Autodesk Inventor part; units mm, degrees
ref_plane "Work Plane1" through (0, 130, 0) normal (0, 1, 0) x (-1, 0, 0)
ref_plane "Work Plane2" through (0, 0, 24.9) normal (0, 0, -1) x (-1, 0, 0)
ref_plane "YZ Plane" through (0, 0, 0) normal (1, 0, 0) x (0, 1, 0)
sketch "Sketch1" plane through (0, 0, 0) normal (0, 0, 1) x (1, 0, 0)
  line L0 (-24.9, 127.5931) -> (-24.9, 125)
  line L1 (-24.9, 125) -> (24.9, 125)
  line L2 (24.9, 125) -> (24.9, 127.5931)
  arc A0 (24.9, 127.5931) -> (-24.9, 127.5931) centre (0, 0) ccw
  point P0 (0, 130)
  dimension "d0" = 130
  dimension "d1" = 5
  dimension "d2" = 49.8
extrude "Extrusion1" add sketch "Sketch1" along normal blind 49.8
chamfer "Chamfer1" distance 5 angle 45 1 edges at (-24.9, 126.2965, 49.8)
ref_plane "Work Plane1" through (0, 130, 0) normal (0, 1, 0) x (-1, 0, 0)
sketch "Sketch2" plane through (0, 130, 0) normal (0, 1, 0) x (-1, 0, 0)
  line L0 (19.9, 49.8) -> (-24.9, 49.8) construction
  line L1 (-24.9, 0) -> (-24.9, 49.8) construction
  line L2 (-24.9, 24.9) -> (31.0612, 24.9) construction
  line L3 (21.9246, 24.9) -> (17.7633, 29.1517)
  line L4 (17.7633, 29.1517) -> (17.7633, 26.5283)
  line L5 (17.7633, 26.5283) -> (13.964, 26.5283)
  line L6 (13.964, 26.5283) -> (13.964, 24.9)
  line L7 (21.9246, 24.9) -> (17.7633, 20.6483)
  line L8 (17.7633, 20.6483) -> (17.7633, 23.2717)
  line L9 (17.7633, 23.2717) -> (13.964, 23.2717)
  line L10 (13.964, 23.2717) -> (13.964, 24.9)
  point P0 (0, 0)
emboss "Emboss1" sketch "Sketch2" operation cut depth 0.8 direction (0, -1, 0)
sketch "Sketch3" plane through (-24.9, 125, 0) normal (0, -1, 0) x (1, 0, 0)
  line L0 (0, 0) -> (49.8, 0)
  line L1 (49.8, 0) -> (49.8, 49.8) construction
  line L2 (49.8, 24.9) -> (6.096, 24.9) construction
  circle A0 centre (18.3, 4.9) radius 3.5
  circle A1 centre (37.55, 4.9) radius 3.5
  circle A2 centre (18.3, 12.4) radius 2.75
  point P0 (24.9, 0)
  dimension "d20" = 7
  dimension "d21" = 7
  dimension "d22" = 20
  dimension "d23" = 20
  dimension "d24" = 12.25
  dimension "d25" = 19.25
  dimension "d26" = 5.5
  dimension "d27" = 12.5
extrude "Extrusion2" cut sketch "Sketch3" against normal blind 2.5
ref_plane "Work Plane2" through (0, 0, 24.9) normal (0, 0, -1) x (-1, 0, 0)
mirror "Mirror1" about plane through (0, 0, 24.9) normal (0, 0, -1) of "Extrusion2"
properties part number "power_signal_socket_cap"
Check sheet for the modelled part. Datum: model origin and axes. Units: mm. A direction names the side the tool comes from. Give positions to 0.01 mm unless a question says otherwise; leave off trailing zeros. Loops run counter-clockwise (first coordinate to the right, second up) from the corner with the lowest first, then second, coordinate; pieces in that order, holes last. Notation, with made-up numbers: M 71,-26 L 104,-26 A17 cw 104,-21 Z; hole C 11.5,61.5 d11. An arc over 180 degrees is marked long. Return JSON: item names as keys, results as strings. Group by question number.
1. Cross-section at A-A on y = 126.25. Record the boundary of the cut face in (x, z), plus the area to 3 significant figures.
2. Thickness scan on L1, parallel to Z at x = -6.6, y = 126.75; L2, parallel to X at y = 126.2, z = 44.5; L3, parallel to X at y = 125.85, z = 44.9. Record the ranges inside material, lowest first.
3. Cross-section at D-D on x = 12.65. Record the boundary of the cut face in (y, z), plus the area to 3 significant figures.
4. Cross-section at C-C on z = 12.4. Record the boundary of the cut face in (x, y).
5. Mould release check, pull along Z, two halves, no side actions. Record for faces 1 (the flat face through (2, 128, 49.8)), 2 (the flat face through (-7, 127.5, 5)), 3 (the flat face through (-24.9, 126, 22)): released by +Z, released by -Z, zero draft, split by the parting line, or undercut.
6. Tool access check on faces 4 (the cylindrical face through (0, 130, 25)), 5 (the flat face through (-15.9, 128.6, 26.528)), 6 (the flat face through (-7, 127.5, 37)). Record the directions out of +Z, -Z, +X, -X, +Y, -Y that give a thin tool (end or side, any length) a straight path to the whole face; none if there is none.
7. Go/stop test with flat-tipped pins: pin 1 (5 mm diameter, centred on x = -6.6, z = 12.4, fed in from -Y); pin 2 (5.5 mm diameter, centred on x = -7.5, z = 43.5, fed in from -Y); pin 3 (8 mm diameter, centred on x = 12.65, z = 4.9, fed in from +Y). Record where each tip stops, or that it passes through.
8. Cross-section at B-B on x = -7.5. Record the boundary of the cut face in (y, z).
Return value:
{
 "1": {"outline": "M -24.9,0 L 24.9,0 L 24.9,49.8 L -19.9,49.8 L -24.9,44.8 Z; hole C -6.6,4.9 d7; hole C -6.6,44.9 d7; hole C -6.6,12.4 d5.5; hole C -6.6,37.4 d5.5; hole C 12.65,4.9 d7; hole C 12.65,44.9 d7", "area": "2,270 mm^2"},
 "2": {"L1": "0 to 1.4, 8.4 to 9.65, 15.15 to 34.65, 40.15 to 41.4, 48.4 to 49.8", "L2": "-24.9 to -10.08, -3.12 to 9.17, 16.13 to 24.9", "L3": "-24.8 to -10.1, -3.1 to 9.15, 16.15 to 24.9"},
 "3": {"outline": "M 125,0 L 129.38,0 L 129.38,49.8 L 125,49.8 L 125,48.4 L 127.5,48.4 L 127.5,41.4 L 125,41.4 L 125,8.4 L 127.5,8.4 L 127.5,1.4 L 125,1.4 Z", "area": "183 mm^2"},
 "4": {"outline": "M -24.9,125 L -9.35,125 L -9.35,127.5 L -3.85,127.5 L -3.85,125 L 24.9,125 L 24.9,127.59 A130 ccw -24.9,127.59 Z"},
 "5": {"face 1": "released by +Z", "face 2": "undercut", "face 3": "zero draft"},
 "6": {"face 4": "+Z, -Z, +Y", "face 5": "+Y", "face 6": "-Y"},
 "7": {"pin 1": "y = 127.5", "pin 2": "y = 125", "pin 3": "y = 129.71"},
 "8": {"outline": "M 125,0 L 129.78,0 L 129.78,49.8 L 125,49.8 L 125,48.28 L 127.5,48.28 L 127.5,41.52 L 125,41.52 L 125,40 L 127.5,40 L 127.5,34.8 L 125,34.8 L 125,15 L 127.5,15 L 127.5,9.8 L 125,9.8 L 125,8.28 L 127.5,8.28 L 127.5,1.52 L 125,1.52 Z"}
}
